Geometry check sheet. Reference: the model listing, model coordinates, mm. Coordinates: 2 decimals unless noted, no trailing zeros. One line per item, written item: value.
Autodesk Inventor part; units mm, degrees
ref_plane "YZ Plane" through (0, 0, 0) normal (1, 0, 0) x (0, 1, 0)
ref_plane "XZ Plane" through (0, 0, 0) normal (0, 1, 0) x (-1, 0, 0)
ref_plane "XY Plane" through (0, 0, 0) normal (0, 0, 1) x (1, 0, 0)
sketch "Sketch1" plane through (0, 0, 0) normal (0, 0, 1) x (1, 0, 0)
  line L0 (0, 0) -> (-6.35, 0)
  line L1 (-6.35, 0) -> (-6.35, 6.35)
  line L2 (-6.35, 6.35) -> (0, 6.35)
  line L3 (0, 6.35) -> (0, 0)
  dimension "d0" = 6.35
  dimension "d1" = 6.35
extrude "Extrusion1" add sketch "Sketch1" along normal blind 76.2
sketch "Sketch2" plane through (0, 0, 0) normal (1, 0, 0) x (0, 0, -1)
  line L0 (-76.2, 0) -> (-76.2, 6.35)
  arc A0 (-76.2, 6.35) -> (-76.2, 0) centre (-76.2, 3.175) ccw
  circle A1 centre (-76.2, 3.175) radius 1.5875
  point P0 (0, 0)
  dimension "d4" = 3.175
  dimension "d5" = 3.175
extrude "Extrusion2" add sketch "Sketch2" against normal blind 6.35 contours A0 L0 A1 | A1 L0 picked at (-76.3266, 2.6612)
extrude "Extrusion3" cut sketch "Sketch2" against normal blind 6.35 contours A1 L0 | L0 A1
(1) Material ranges on probe 1 along Y at (x, z) = (-2.75, 76.2); probe 2 along Z at (x, y) = (-5.25, 2); probe 3 along Z at (x, y) = (-3.25, 2.5), recorded low to high. Write a range as from..to.
Reply:
probe 1: 0..1.59, 4.76..6.35
probe 2: 0..75.13, 77.27..79.15
probe 3: 0..74.76, 77.64..79.3
(2) Release check for a two-part mould opening along Z. For faces 1 (the face through (-3, 3, 0)), 2 (the face through (-3, 6.35, 38)), 3 (the face through (-3.131, 4.514, 75.347)) record: pulls with the +Z half, pulls with the -Z half, needs draft (parallel to the pull), parting line crosses it, or undercut.
Reply:
face 1: pulls with the -Z half
face 2: needs draft
face 3: undercut
(3) Go/stop test with flat-tipped pins: pin 1 Ø1 at (y, z) = (3, 10) entering from +X; pin 2 Ø1 at (x, y) = (-0.5, 4.5) entering from +Z. Record where each tip stops, or that it passes through.
Reply:
pin 1: x = 0
pin 2: z = 79.27
